Geometry check sheet. Reference: the model listing, model coordinates, mm. A direction names the side the tool comes from. Coordinates: 2 decimals unless noted, no trailing zeros. Order: outer loops, then holes, each group sorted by start corner. A loop starts at its lowest first (then second) coordinate and runs counter-clockwise, first axis right, second up. Notation, with made-up numbers: (0, -4) -> (7, -4) arc R23 ccw to (7, 10) -> close; hole circle Ø2 at (-33, 55). An arc over 180 degrees is marked (long way). Answer in a Markdown table with one row per item. Add a question column.
Autodesk Inventor part; units mm, degrees
ref_plane "YZ Plane" through (0, 0, 0) normal (1, 0, 0) x (0, 1, 0)
ref_plane "XZ Plane" through (0, 0, 0) normal (0, 1, 0) x (-1, 0, 0)
ref_plane "XY Plane" through (0, 0, 0) normal (0, 0, 1) x (1, 0, 0)
sketch "Sketch1" plane through (0, 0, 0) normal (0, 0, 1) x (1, 0, 0)
  circle A0 centre (0, 0) radius 17.4625
  circle A1 centre (0, 0) radius 7.9375
  dimension "d0" = 34.925
  dimension "d2" = 15.875
extrude "Extrusion1" add sketch "Sketch1" along normal blind 4.3656
sketch "Sketch2" plane through (0, 0, 4.3656) normal (0, 0, 1) x (1, 0, 0)
  circle A0 centre (0, 0) radius 17.4625
  circle A1 centre (0, 0) radius 9.525
  circle A2 centre (0, 0) radius 14.2875
  dimension "d5" = 19.05
  dimension "d8" = 28.575
extrude "Extrusion2" cut sketch "Sketch2" against normal blind 0.5953 contours A2
chamfer "Chamfer1" distance 0.3969 angle 45 3 edges at (-17.4625, 0, 4.3656) (-9.525, 0, 4.3656) (-14.2875, 0, 4.3656)
mirror "Mirror1" about plane through (0, 0, 0) normal (0, 0, -1)
properties part number "R10-2RS"
(1) Scan lines: line 1 along Y through (x, z) = (0, -3.85) (1 decimal); line 2 along Z through (x, y) = (-11.5, -8); line 3 along Y through (x, z) = (0, -1.5). Record each from-to range of solid material in increasing order.
(2) Cross-section at A-A (z = 1.5). Enter the section's corners in (x, y) (1 decimal), plus the area to 3 significant figures.
(3) Access from +Z, -Z, +X, -X, +Y, -Y to the whole of each face (thin tool, end or side, straight path). Record for faces 1 (the face through (-3, -9.3, -3.77)), 2 (the face through (-1.72, -7.75, 0.06)).
(4) Mould release check, pull along Y, two halves, no side actions. Record for faces 3 (the face through (-13.858, 10.626, -0.056)), 4 (the face through (0, 8.2, 4.366)), 5 (the face through (3, -9.3, 3.77)): +Y half, -Y half, draft (parallel to the pull), parting line (faces both ways), or undercut.
(5) Go/stop test with flat-tipped pins: P1, Ø2, axis at x = 2.5, y = -10, coming from the -Z side; P2, Ø4, axis at x = 3, z = -1, coming from the -Y side; P3, Ø2, axis at x = 3.5, z = -3.5, coming from the -Y side. Record where each tip stops, or that it passes through.
Checks:
| question | item | result |
|---|---|---|
| 1 | line 1 | -17.5 to -14.3, -9.5 to -7.9, 7.9 to 9.5, 14.3 to 17.5 |
| 1 | line 2 | -3.77 to 3.77 |
| 1 | line 3 | -17.46 to -7.94, 7.94 to 17.46 |
| 2 | outline | circle Ø34.9 at (0, 0); hole circle Ø15.9 at (0, 0) |
| 2 | area | 760 mm² |
| 3 | face 1 | -Z |
| 3 | face 2 | +Z, -Z |
| 4 | face 3 | parting line |
| 4 | face 4 | draft |
| 4 | face 5 | undercut |
| 5 | P1 | z = -4.19 |
| 5 | P2 | y = -17.43 |
| 5 | P3 | y = -17.28 |
